from build123d import *

# Parameters (mm, degrees)
EXTRUDE_1_DEPTH        = 3
CUT_EXTRUDE_1_REACH    = 69.785
SKETCH_3_R             = 3.25
CUT_EXTRUDE_2_DEPTH    = 0.8
CUT_EXTRUDE_START      = -2.2
SKETCH_3_2_R           = 3.25
CUT_EXTRUDE_3_DEPTH    = 0.8
PATTERN_LINEAR_1_COUNT = 2
PATTERN_LINEAR_1_PITCH = 63.6
CUT_EXTRUDE_4_DEPTH    = 0.8
SKETCH_5_W             = 55.6
SKETCH_5_H             = 4
CUT_EXTRUDE_5_DEPTH    = 0.8


with BuildPart() as part:
    # 草图1 → 凸台-拉伸1 (new body)
    with BuildSketch(Plane.XY):
        with BuildLine():
            Line((0, 4), (63.6, 4))
            ThreePointArc((63.6, 4), (67.6, 0), (63.6, -4))
            Line((63.6, -4), (0, -4))
            ThreePointArc((0, -4), (-4, 0), (0, 4))
        make_face()
    extrude(amount=-EXTRUDE_1_DEPTH)

    # 草图2 → 切除-拉伸1 (cut, up to next)
    with BuildSketch(Plane.XY, mode=Mode.PRIVATE) as cut_extrude_1_sk1:
        with BuildLine():
            Line((1.322875656, -1.5), (2.883140649, -1.5))
            ThreePointArc((2.883140649, -1.5), (3.25, 0), (2.883140649, 1.5))
            Line((2.883140649, 1.5), (1.322875656, 1.5))
            ThreePointArc((1.322875656, 1.5), (0, 2), (-1.322875656, 1.5))
            Line((-1.322875656, 1.5), (-2.883140649, 1.5))
            ThreePointArc((-2.883140649, 1.5), (-3.25, 0), (-2.883140649, -1.5))
            Line((-2.883140649, -1.5), (-1.322875656, -1.5))
            ThreePointArc((-1.322875656, -1.5), (0, -2), (1.322875656, -1.5))
        make_face()
    cut_extrude_1_tool1 = extrude(cut_extrude_1_sk1.sketch, amount=-CUT_EXTRUDE_1_REACH, mode=Mode.PRIVATE) & part.part
    cut_extrude_1 = cut_extrude_1_tool1.solids().sort_by_distance((0, 0, 0))[0]
    add(cut_extrude_1, mode=Mode.SUBTRACT)

    # 草图3 → 切除-拉伸2 (cut)
    with BuildSketch(Plane.XY):
        Circle(SKETCH_3_R)
    cut_extrude_2 = extrude(amount=-CUT_EXTRUDE_2_DEPTH, mode=Mode.SUBTRACT)

    # 草图3<2> → 切除-拉伸3 (cut)
    with BuildSketch(Plane.XY.offset(CUT_EXTRUDE_START)):
        Circle(SKETCH_3_2_R)
    cut_extrude_3 = extrude(amount=-CUT_EXTRUDE_3_DEPTH, mode=Mode.SUBTRACT)

    # 阵列(线性)1: 切除-拉伸1, 切除-拉伸2, 切除-拉伸3 ×2
    with Locations(*[(i * PATTERN_LINEAR_1_PITCH, 0, 0) for i in range(1, PATTERN_LINEAR_1_COUNT)]):
        add(cut_extrude_1, mode=Mode.SUBTRACT)
        add(cut_extrude_2, mode=Mode.SUBTRACT)
        add(cut_extrude_3, mode=Mode.SUBTRACT)

    # 草图4 → 切除-拉伸4 (cut)
    with BuildSketch(Plane.XY):
        with BuildLine():
            Line((3.464101615, 2), (60.135898385, 2))
            ThreePointArc((60.135898385, 2), (59.6, 0), (60.135898385, -2))
            Line((60.135898385, -2), (3.464101615, -2))
            ThreePointArc((3.464101615, -2), (4, 0), (3.464101615, 2))
        make_face()
    extrude(amount=-CUT_EXTRUDE_4_DEPTH, mode=Mode.SUBTRACT)

    # 草图5 → 切除-拉伸5 (cut)
    with BuildSketch(Plane(origin=(0, 0, -3), x_dir=(-1, 0, 0), z_dir=(0, 0, -1))):
        with Locations((-31.8, 0)):
            Rectangle(SKETCH_5_W, SKETCH_5_H)
    extrude(amount=-CUT_EXTRUDE_5_DEPTH, mode=Mode.SUBTRACT)


solid = part.part
Input: part model. Units: mm. Frame: model coordinates. A direction names the side the tool comes from. Coordinates: 2 decimals unless noted, no trailing zeros. Order: outer loops, then holes, each group sorted by start corner. A loop starts at its lowest first (then second) coordinate and runs counter-clockwise, first axis right, second up. Notation, with made-up numbers: M 12.5,49 L 42.5,49 A18 cw 42.5,71 Z; hole C 71.5,86.5 d1. An arc over 180 degrees is marked long. Write item = value, one per line. Start each with the question number.
(1) First-contact query: P1, Ø1.1, axis at x = 66, z = -1.5, coming from the -Y side; P2, Ø1, axis at x = 16.5, y = 1, coming from the -Z side; P3, Ø0.5, axis at x = -1, y = -2, coming from the +Z side. Flat tips, straight axial feed; report the tip coordinate or a pass-through.
(2) Reachability of faces 1 (the flat face through (0, 2.4, -2.2)), 2 (the flat face through (61, -1.5, -1)), 3 (the flat face through (0, 2.4, -0.8)) from +Z, -Z, +X, -X, +Y, -Y: full face, straight path, thin tool, end or side. Return the list, or none.
(3) Section C-C on x = 30. Output: boundary loops of the cut face in (y, z).
(4) Pull-direction query (X, two-part tool) for faces 4 (the flat face through (32, 3, -3)), 5 (the flat face through (-2, 1.5, -1)), 6 (the flat face through (66, -1.5, -1)); classes: released by +X, released by -X, zero draft, split by the parting line, or undercut.
(5) Section A-A on y = 0. Output: boundary loops of the cut face in (x, z).
(6) Section B-B on z = -1.7. Output: boundary loops of the cut face in (x, y).
(7) Line query: line 1 along X through (y, z) = (-0.25, -2); line 2 along X through (y, z) = (-0.25, -0.35); line 3 along Y through (x, z) = (49.5, -0.4). Output: solid intervals per line, ascending. Write a range as [from, to].
Result set:
q1.P1 = -3.55
q1.P2 = -2.2
q1.P3 = -0.8
q2.face_1 = -Z
q2.face_2 = +Z, -Z
q2.face_3 = +Z
q3.outline = M -4,-3 L -2,-3 L -2,-2.2 L 2,-2.2 L 2,-3 L 4,-3 L 4,0 L 2,0 L 2,-0.8 L -2,-0.8 L -2,0 L -4,0 Z
q4.face_4 = zero draft
q4.face_5 = undercut
q4.face_6 = undercut
q5.outline = M -4,-3 L -3.25,-3 L -3.25,0 L -4,0 Z; M 3.25,-3 L 4,-3 L 4,-2.2 L 59.6,-2.2 L 59.6,-3 L 60.35,-3 L 60.35,0 L 59.6,0 L 59.6,-0.8 L 4,-0.8 L 4,0 L 3.25,0 Z; M 66.85,-3 L 67.6,-3 L 67.6,0 L 66.85,0 Z
q6.outline = M 0,-4 L 63.6,-4 A4 ccw 63.6,4 L 0,4 A4 ccw Z; hole M -2.88,-1.5 L -1.32,-1.5 A2 ccw 1.32,-1.5 L 2.88,-1.5 A3.25 ccw 2.88,1.5 L 1.32,1.5 A2 ccw -1.32,1.5 L -2.88,1.5 A3.25 ccw Z; hole M 60.72,-1.5 L 62.28,-1.5 A2 ccw 64.92,-1.5 L 66.48,-1.5 A3.25 ccw 66.48,1.5 L 64.92,1.5 A2 ccw 62.28,1.5 L 60.72,1.5 A3.25 ccw Z
q7.line_1 = [-3.99, -3.24], [3.24, 60.36], [66.84, 67.59]
q7.line_2 = [-3.99, -3.24], [3.24, 3.99], [59.61, 60.36], [66.84, 67.59]
q7.line_3 = [-4, -2], [2, 4]
